from build123d import *

# Parameters (mm, degrees)
SKETCH1_W           = 19.5
SKETCH1_H           = 26
BOSS_EXTRUDE1_DEPTH = 10
CUT_EXTRUDE1_REACH  = 21.08
SKETCH2_W           = 15.6
SKETCH2_H           = 20.8
CUT_EXTRUDE2_REACH  = 31.514
SKETCH3_R           = 1.25
CUT_EXTRUDE5_DEPTH  = 10
SKETCH8_W           = 19.5
SKETCH8_H           = 10
BOSS_EXTRUDE2_DEPTH = 1.4875
SKETCH9_W           = 15.6
SKETCH9_H           = 1.4875
SKETCH9_W_2         = 1.95
CUT_EXTRUDE7_DEPTH  = 21.123373381
SKETCH10_W          = 1.95
SKETCH10_H          = 10
BOSS_EXTRUDE3_DEPTH = 14.2875
BOSS_EXTRUDE4_DEPTH = 2.55


with BuildPart() as part:
    # Sketch1 → Boss-Extrude1 (new body)
    with BuildSketch(Plane.XY):
        Rectangle(SKETCH1_W, SKETCH1_H)
    extrude(amount=BOSS_EXTRUDE1_DEPTH)

    # Sketch2 → Cut-Extrude1 (cut, up to next)
    with BuildSketch(Plane.XY.offset(10), mode=Mode.PRIVATE) as cut_extrude1_sk1:
        Rectangle(SKETCH2_W, SKETCH2_H)
    cut_extrude1_tool1 = extrude(cut_extrude1_sk1.sketch, amount=-CUT_EXTRUDE1_REACH, mode=Mode.PRIVATE) & part.part
    add(cut_extrude1_tool1.solids().sort_by_distance((0, 0, 10))[0], mode=Mode.SUBTRACT)

    # Sketch3 → Cut-Extrude2 (cut, up to next)
    with BuildSketch(Plane.XZ.offset(13), mode=Mode.PRIVATE) as cut_extrude2_sk1:
        with Locations(Location((-5.85, 5, 0), (0, 0, 270))):
            Circle(SKETCH3_R)
    cut_extrude2_tool1 = extrude(cut_extrude2_sk1.sketch, amount=-CUT_EXTRUDE2_REACH, mode=Mode.PRIVATE) & part.part
    # Sketch3 → Cut-Extrude2 (cut, up to next)
    with BuildSketch(Plane.XZ.offset(13), mode=Mode.PRIVATE) as cut_extrude2_sk2:
        with Locations(Location((5.85, 5, 0), (0, 0, 270))):
            Circle(SKETCH3_R)
    cut_extrude2_tool2 = extrude(cut_extrude2_sk2.sketch, amount=-CUT_EXTRUDE2_REACH, mode=Mode.PRIVATE) & part.part
    add(cut_extrude2_tool1.solids().sort_by_distance((-5.85, -13, 5))[0], mode=Mode.SUBTRACT)
    add(cut_extrude2_tool2.solids().sort_by_distance((5.85, -13, 5))[0], mode=Mode.SUBTRACT)

    # Sketch6 → Cut-Extrude5 (cut)
    with BuildSketch(Plane.XY.offset(10)):
        Polygon((-7.8, -1.2875), (-9.75, -1.2875), (-9.75, -13), (9.75, -13), (9.75, -1.2875), (7.8, -1.2875), (7.8, -10.4), (-7.8, -10.4), align=None)
    extrude(amount=-CUT_EXTRUDE5_DEPTH, mode=Mode.SUBTRACT)

    # Sketch8 → Boss-Extrude2 (add)
    with BuildSketch(Plane(origin=(0, 13, 0), x_dir=(1, 0, 0), z_dir=(0, 1, 0))):
        with Locations((0, -5)):
            Rectangle(SKETCH8_W, SKETCH8_H)
    extrude(amount=BOSS_EXTRUDE2_DEPTH)

    # Sketch9 → Cut-Extrude7 (cut, through all)
    with BuildSketch(Plane.XY.offset(10)):
        with Locations((0, -0.54375)):
            Rectangle(SKETCH9_W, SKETCH9_H)
        with Locations((8.775, -0.54375)):
            Rectangle(SKETCH9_W_2, SKETCH9_H)
        with Locations((-8.775, -0.54375)):
            Rectangle(SKETCH9_W_2, SKETCH9_H)
    extrude(amount=-CUT_EXTRUDE7_DEPTH, mode=Mode.SUBTRACT)

    # Sketch10 → Boss-Extrude3 (add)
    with BuildSketch(Plane.XZ.offset(-0.2)):
        with Locations((-8.775, 5)):
            Rectangle(SKETCH10_W, SKETCH10_H)
        with Locations((8.775, 5)):
            Rectangle(SKETCH10_W, SKETCH10_H)
    extrude(amount=BOSS_EXTRUDE3_DEPTH)

    # Sketch11 → Boss-Extrude4 (add)
    with BuildSketch(Plane.XY.offset(10)):
        Polygon((-9.75, -14.0875), (-9.75, 14.4875), (9.75, 14.4875), (9.75, -14.0875), (7.8, -14.0875), (7.8, 10.4), (-7.8, 10.4), (-7.8, -14.0875), align=None)
    extrude(amount=BOSS_EXTRUDE4_DEPTH)


solid = part.part
The listing builds one solid part. Answer for the finished solid, in the listing's coordinates (mm). A direction names the side the tool comes from. Coordinates: 2 decimals unless noted, no trailing zeros. Loops run counter-clockwise (first coordinate to the right, second up) from the corner with the lowest first, then second, coordinate; pieces in that order, holes last. Notation, with made-up numbers: (46, 11.25) -> (56, 11.25) arc R22 ccw to (56, 18.25) -> close; hole circle Ø4 at (44, 4). An arc over 180 degrees is marked (long way). Write item = value, one per line. Start each with the question number.
1) The mould has two halves that part along X. Classify faces 3 (the face through (9.75, 0, 6)), 4 (the face through (7.8, -2, 6)), 5 (the face through (-7.8, -2, 6)), 6 (the face through (0, 11, 12.55)): released by +X, released by -X, zero draft, split by the parting line, or undercut.
2) A tool of negligible diameter and unlimited length cuts with its end or side. For faces 1 (the face through (-9, -14.088, 6)), 2 (the face through (0, 10.4, 6)), from which of +Z, -Z, +X, -X, +Y, -Y can it reach the whole face along a straight path? Write none if from no direction.
3) A cutting plane is placed at B-B (z = 3). Give the vertices of the cut face in (x, y).
4) A cutting plane is placed at A-A (y = 0). Give the vertices of the cut face in (x, z).
5) A cutting plane is placed at C-C (x = 3.25). Give the vertices of the cut face in (y, z).
6) Straight lines are drawn through the part: line 1 (X direction, y = -7, z = 7.75); line 2 (Y direction, x = -7.25, z = 7). For each, find the intervals that lie inside material, in ascending order. Write a range as from..to.
Responses:
q1.face_3 = released by +X
q1.face_4 = undercut
q1.face_5 = undercut
q1.face_6 = zero draft
q2.face_1 = +Z, -Z, +X, -X, -Y
q2.face_2 = +Z, -Z, -Y
q3.outline = (-9.75, -14.09) -> (-7.8, -14.09) -> (-7.8, 10.4) -> (7.8, 10.4) -> (7.8, -14.09) -> (9.75, -14.09) -> (9.75, 14.49) -> (-9.75, 14.49) -> close
q4.outline = (-9.75, 0) -> (-7.8, 0) -> (-7.8, 12.55) -> (-9.75, 12.55) -> close; (7.8, 0) -> (9.75, 0) -> (9.75, 12.55) -> (7.8, 12.55) -> close
q5.outline = (10.4, 0) -> (14.49, 0) -> (14.49, 12.55) -> (10.4, 12.55) -> close
q6.line_1 = -9.75..-7.8, 7.8..9.75
q6.line_2 = 10.4..14.49
